from build123d import *

# Parameters (mm, degrees)
F0_R     = 34.75
F1_DEPTH = 49
F3_DEPTH = 21
F4_R     = 31.8
F5_DEPTH = 8
F6_R     = 31.8
F7_DEPTH = 8


with BuildPart() as f1:
    # F0 (on Top) → F1 (new body)
    with BuildSketch(Plane.XY):
        Circle(F0_R)
    extrude(amount=F1_DEPTH)

    # F2 (on face) → F3 (join)
    with BuildSketch(Plane.XY.offset(49)):
        with BuildLine():
            Line((-2.639753, 28.010705), (-2.639753, 34.649592))
            ThreePointArc((-2.639753, 34.649592), (-5.436098, 34.32217), (-8.196759, 33.769448))
            Line((-8.196759, 33.769448), (-6.14523, 27.455492))
            Line((-6.14523, 27.455492), (-11.166338, 25.824036))
            Line((-11.166338, 25.824036), (-13.217867, 32.137992))
            ThreePointArc((-13.217867, 32.137992), (-15.77617, 30.962477), (-18.230914, 29.583716))
            Line((-18.230914, 29.583716), (-14.328675, 24.212744))
            Line((-14.328675, 24.212744), (-18.599884, 21.109529))
            Line((-18.599884, 21.109529), (-22.502124, 26.480501))
            ThreePointArc((-22.502124, 26.480501), (-24.571961, 24.571961), (-26.480501, 22.502124))
            Line((-26.480501, 22.502124), (-21.109529, 18.599884))
            Line((-21.109529, 18.599884), (-24.212744, 14.328675))
            Line((-24.212744, 14.328675), (-29.583716, 18.230914))
            ThreePointArc((-29.583716, 18.230914), (-30.962477, 15.77617), (-32.137992, 13.217867))
            Line((-32.137992, 13.217867), (-25.824036, 11.166338))
            Line((-25.824036, 11.166338), (-27.455492, 6.14523))
            Line((-27.455492, 6.14523), (-33.769448, 8.196759))
            ThreePointArc((-33.769448, 8.196759), (-34.32217, 5.436098), (-34.649592, 2.639753))
            Line((-34.649592, 2.639753), (-28.010705, 2.639753))
            Line((-28.010705, 2.639753), (-28.010705, -2.639753))
            Line((-28.010705, -2.639753), (-34.649592, -2.639753))
            ThreePointArc((-34.649592, -2.639753), (-34.32217, -5.436098), (-33.769448, -8.196759))
            Line((-33.769448, -8.196759), (-27.455492, -6.14523))
            Line((-27.455492, -6.14523), (-25.824036, -11.166338))
            Line((-25.824036, -11.166338), (-32.137992, -13.217867))
            ThreePointArc((-32.137992, -13.217867), (-30.962477, -15.77617), (-29.583716, -18.230914))
            Line((-29.583716, -18.230914), (-24.212744, -14.328675))
            Line((-24.212744, -14.328675), (-21.109529, -18.599884))
            Line((-21.109529, -18.599884), (-26.480501, -22.502124))
            ThreePointArc((-26.480501, -22.502124), (-24.571961, -24.571961), (-22.502124, -26.480501))
            Line((-22.502124, -26.480501), (-18.599884, -21.109529))
            Line((-18.599884, -21.109529), (-14.328675, -24.212744))
            Line((-14.328675, -24.212744), (-18.230914, -29.583716))
            ThreePointArc((-18.230914, -29.583716), (-15.77617, -30.962477), (-13.217867, -32.137992))
            Line((-13.217867, -32.137992), (-11.166338, -25.824036))
            Line((-11.166338, -25.824036), (-6.14523, -27.455492))
            Line((-6.14523, -27.455492), (-8.196759, -33.769448))
            ThreePointArc((-8.196759, -33.769448), (-5.436098, -34.32217), (-2.639753, -34.649592))
            Line((-2.639753, -34.649592), (-2.639753, -28.010705))
            Line((-2.639753, -28.010705), (2.639753, -28.010705))
            Line((2.639753, -28.010705), (2.639753, -34.649592))
            ThreePointArc((2.639753, -34.649592), (5.436098, -34.32217), (8.196759, -33.769448))
            Line((8.196759, -33.769448), (6.14523, -27.455492))
            Line((6.14523, -27.455492), (11.166338, -25.824036))
            Line((11.166338, -25.824036), (13.217867, -32.137992))
            ThreePointArc((13.217867, -32.137992), (15.77617, -30.962477), (18.230914, -29.583716))
            Line((18.230914, -29.583716), (14.328675, -24.212744))
            Line((14.328675, -24.212744), (18.599884, -21.109529))
            Line((18.599884, -21.109529), (22.502124, -26.480501))
            ThreePointArc((22.502124, -26.480501), (24.571961, -24.571961), (26.480501, -22.502124))
            Line((26.480501, -22.502124), (21.109529, -18.599884))
            Line((21.109529, -18.599884), (24.212744, -14.328675))
            Line((24.212744, -14.328675), (29.583716, -18.230914))
            ThreePointArc((29.583716, -18.230914), (30.962477, -15.77617), (32.137992, -13.217867))
            Line((32.137992, -13.217867), (25.824036, -11.166338))
            Line((25.824036, -11.166338), (27.455492, -6.14523))
            Line((27.455492, -6.14523), (33.769448, -8.196759))
            ThreePointArc((33.769448, -8.196759), (34.32217, -5.436098), (34.649592, -2.639753))
            Line((34.649592, -2.639753), (28.010705, -2.639753))
            Line((28.010705, -2.639753), (28.010705, 2.639753))
            Line((28.010705, 2.639753), (34.649592, 2.639753))
            ThreePointArc((34.649592, 2.639753), (34.32217, 5.436098), (33.769448, 8.196759))
            Line((33.769448, 8.196759), (27.455492, 6.14523))
            Line((27.455492, 6.14523), (25.824036, 11.166338))
            Line((25.824036, 11.166338), (32.137992, 13.217867))
            ThreePointArc((32.137992, 13.217867), (30.962477, 15.77617), (29.583716, 18.230914))
            Line((29.583716, 18.230914), (24.212744, 14.328675))
            Line((24.212744, 14.328675), (21.109529, 18.599884))
            Line((21.109529, 18.599884), (26.480501, 22.502124))
            ThreePointArc((26.480501, 22.502124), (24.571961, 24.571961), (22.502124, 26.480501))
            Line((22.502124, 26.480501), (18.599884, 21.109529))
            Line((18.599884, 21.109529), (14.328675, 24.212744))
            Line((14.328675, 24.212744), (18.230914, 29.583716))
            ThreePointArc((18.230914, 29.583716), (15.77617, 30.962477), (13.217867, 32.137992))
            Line((13.217867, 32.137992), (11.166338, 25.824036))
            Line((11.166338, 25.824036), (6.14523, 27.455492))
            Line((6.14523, 27.455492), (8.196759, 33.769448))
            ThreePointArc((8.196759, 33.769448), (5.436098, 34.32217), (2.639753, 34.649592))
            Line((2.639753, 34.649592), (2.639753, 28.010705))
            Line((2.639753, 28.010705), (-2.639753, 28.010705))
        make_face()
    extrude(amount=F3_DEPTH)

    # F4 (on face) → F5 (join)
    with BuildSketch(Plane.XY.offset(70)):
        Circle(F4_R)
    extrude(amount=F5_DEPTH)

    # F6 (on face) → F7 (cut)
    with BuildSketch(Plane(origin=(0, 0, 0), x_dir=(1, 0, 0), z_dir=(0, 0, -1))):
        Circle(F6_R)
    extrude(amount=-F7_DEPTH, mode=Mode.SUBTRACT)


solid = f1.part
Can you work these out from the model? Positions are in its coordinate system, mm. A direction names the side the tool comes from. Coordinates: 2 decimals unless noted, no trailing zeros. Write each loop counter-clockwise with the first axis right and the second up, starting at its lowest first coordinate (ties: lowest second). Pieces come first, ordered by that corner, then holes. Notation, with made-up numbers: (-27.75, -8) -> (23.25, -8) arc R15 ccw to (23.25, 11) -> close; hole circle Ø9 at (68, 11.5). An arc over 180 degrees is marked (long way). Write each question's results on one line, items separated by ' | '. Start each with the question number.
Q1. We'd pull the mould along Z, two halves only. Please class faces 1 (the face through (-24.544, 24.6, 59.353)), 2 (the face through (5, -33, 70)), 3 (the face through (26.94, 16.31, 59.35)): +Z half, -Z half, draft (parallel to the pull), parting line (faces both ways), or undercut.
Q2. If I drill on probe 1 along X at (y, z) = (29.5, 65); probe 2 along Y at (x, z) = (0, 5); probe 3 along X at (y, z) = (-18, 68.5), over which ranges is the centre line in solid material (lowest first)?
Q3. Imagine slicing it at C-C (z = 45.5). Write out the boundary of the cut face in (x, y), then the cut area to 3 significant figures.
Q4. On a 3-axis mill with a long thin cutter (end or side, diameter ignored), from which of +Z, -Z, +X, -X, +Y, -Y can I reach the whole of each face in a straight line? I mean faces 4 (the face through (12.2, 29, 59.4)), 5 (the face through (16.25, 26.86, 59.35)), 6 (the face through (31, 0, 49)). Say none if no direction works.
Q5. I'm going to push flat-ended pins straight in: pin 1 (5 mm diameter, centred on x = -21, y = 10, fed in from -Z); pin 2 (1.8 mm diameter, centred on x = -5.5, y = 33.5, fed in from +Z); pin 3 (7.5 mm diameter, centred on y = -32.5, z = 57, fed in from -X). Where does each tip first touch, or does it pass through?
Q6. Imagine slicing it at A-A (y = 0). Write out the boundary of the cut face in (x, z).
Taken from the geometry:
1) face 1: draft | face 2: +Z half | face 3: undercut
2) probe 1: x = -18.17 to -12.36, -6.81 to -2.64, 2.64 to 6.81, 12.36 to 18.17 | probe 2: y = -34.75 to -31.8, 31.8 to 34.75 | probe 3: x = -29.72 to -29.27, -21.55 to 21.55, 29.27 to 29.72
3) outline: circle Ø69.5 at (0, 0) | area: 3,790 mm^2
4) face 4: +Y | face 5: none | face 6: +X
5) pin 1: stops at z = 8 | pin 2: stops at z = 70 | pin 3: stops at x = -18.23
6) outline: (-34.75, 0) -> (-31.8, 0) -> (-31.8, 8) -> (31.8, 8) -> (31.8, 0) -> (34.75, 0) -> (34.75, 49) -> (28.01, 49) -> (28.01, 70) -> (31.8, 70) -> (31.8, 78) -> (-31.8, 78) -> (-31.8, 70) -> (-28.01, 70) -> (-28.01, 49) -> (-34.75, 49) -> close
